Check sheet for the modelled part. Datum: model origin and axes. Units: mm. A direction names the side the tool comes from. Give positions to 0.01 mm unless a question says otherwise; leave off trailing zeros. Order: outer loops, then holes, each group sorted by start corner. A loop starts at its lowest first (then second) coordinate and runs counter-clockwise, first axis right, second up.
Item 1: Release check for a two-part mould opening along Z. For faces 1 (the flat face through (38.348, 6.674, 45.143)), 2 (the flat face through (62.992, 3, 20)), 3 (the flat face through (31.212, 2.655, 1.252)) record: released by +Z, released by -Z, zero draft, split by the parting line, or undercut.
Item 2: Sectioned sample at D-D on z = 4. Record the boundary of the cut face in (x, y), and give its area (3 significant figures).
Item 3: Sectioned sample at A-A on y = 8.5. Record the boundary of the cut face in (x, z).
Item 4: Sectioned sample at B-B on x = 48.5. Record the boundary of the cut face in (y, z).
Item 5: Material ranges on line 1 along X through (y, z) = (3.5, 41.5); line 2 along X through (y, z) = (10.5, 5); line 3 along Y through (x, z) = (21, 32), recorded low to high.
Item 6: Sectioned sample at C-C on z = 40.5. Record the boundary of the cut face in (x, y), and give its area (3 significant figures).
Item 7: Gauge pin test, flat ends, axial feed: P1, Ø1, axis at x = 41, z = 6, coming from the +Y side; P2, Ø3.5, axis at x = 57.404, y = 5.588, coming from the +Z side; P3, Ø3.5, axis at x = 5.588, y = 5.588, coming from the -Z side. Record the tip position at first contact, or that the pin passes through.
Item 8: Access from +Z, -Z, +X, -X, +Y, -Y to the whole of each face (thin tool, end or side, straight path). Record for faces 4 (the flat face through (31.055, 3.398, 47.084)), 5 (the flat face through (31, 2, 0)), 6 (the cylindrical face through (7.37, 6.33, 3.13)).
from build123d import *

# Parameters (mm, degrees)
F1_DEPTH = 62.992
F2_T     = -2.54
F3_W     = 11.176
F3_H     = 11.176
F3_R     = 1.9304
F4_DEPTH = 6.35


with BuildPart() as f1:
    # F0 (on Right) → F1 (new body)
    with BuildSketch(Plane.YZ):
        with BuildLine():
            Line((0, 34.29), (0, 0))
            Line((0, 0), (2.54, 0))
            Line((2.54, 0), (2.54, 34.29))
            ThreePointArc((2.54, 34.29), (3.0543819704, 40.5698861973), (4.5838156026, 46.6823646004))
            Line((4.5838156026, 46.6823646004), (2.1783345915, 47.498))
            ThreePointArc((2.1783345915, 47.498), (0.5482373448, 40.9832130848), (0, 34.29))
        make_face()
        with BuildLine():
            Line((2.54, 34.29), (2.54, 0))
            Line((2.54, 0), (7.3968325046, 53.0323646004))
            ThreePointArc((7.3968325046, 53.0323646004), (5.8471852484, 49.920774345), (4.5838156026, 46.6823646004))
            ThreePointArc((4.5838156026, 46.6823646004), (3.0543819704, 40.5698861973), (2.54, 34.29))
        make_face()
    extrude(amount=F1_DEPTH)

    # F2
    f2_openings = [f1.faces().sort_by_distance(p)[0] for p in [
        (31.496, 4.968416, 26.516182),
    ]]
    offset(amount=F2_T, openings=f2_openings, kind=Kind.INTERSECTION)

    # F3 (on face) → F4 (join)
    with BuildSketch(Plane(origin=(0, 0, 0), x_dir=(1, 0, 0), z_dir=(0, 0, -1))):
        with Locations((57.404, -5.588)):
            Rectangle(F3_W, F3_H)
        with Locations((57.404, -5.588)):
            Circle(F3_R, mode=Mode.SUBTRACT)
        with Locations((5.588, -5.588)):
            Rectangle(F3_W, F3_H)
        with Locations((5.588, -5.588)):
            Circle(F3_R, mode=Mode.SUBTRACT)
    extrude(amount=-F4_DEPTH)


solid = f1.part
Report:
1. face 1: undercut
1. face 2: zero draft
1. face 3: released by -Z
2. outline: (0, 0) - (62.99, 0) - (62.99, 11.18) - (51.82, 11.18) - (51.82, 2.54) - (11.18, 2.54) - (11.18, 11.18) - (0, 11.18) - close; hole circle Ø3.86 at (5.59, 5.59); hole circle Ø3.86 at (57.4, 5.59)
2. area: 330 mm2
3. outline: (0, 0) - (11.18, 0) - (11.18, 6.35) - (0, 6.35) - close; (51.82, 0) - (62.99, 0) - (62.99, 6.35) - (51.82, 6.35) - close
4. outline: (0, 0) - (2.54, 0) - (2.77, 2.54) - (2.54, 2.54) - (2.54, 34.29) arc R38.59 cw to (3.85, 44.25) - (6.26, 43.43) arc R36.05 cw to (6.64, 44.79) - (7.4, 53.03) arc R38.59 ccw to (4.58, 46.68) - (2.18, 47.5) arc R41.13 ccw to (0, 34.29) - close
5. line 1: x = 0 to 2.54, 60.45 to 62.99
5. line 2: x = 0 to 11.18, 51.82 to 62.99
5. line 3: y = 0 to 2.54
6. outline: (0, 0.47) - (62.99, 0.47) - (62.99, 6.25) - (60.45, 6.25) - (60.45, 3.04) - (2.54, 3.04) - (2.54, 6.25) - (0, 6.25) - close
6. area: 178 mm2
7. P1: stops at y = 2.54
7. P2: stops at z = 52.93
7. P3: stops at z = 43.43
8. face 4: +Z, +X, -X
8. face 5: -Z, +X, -X, +Y, -Y
8. face 6: -Z
